Could you check a few things on this model? Use its own coordinates, in mm. Face numbers are marked on the shaded views. Give positions to 0.01 mm unless a question says otherwise; leave off trailing zeros. Loops run counter-clockwise (first coordinate to the right, second up) from the corner with the lowest first, then second, coordinate; pieces in that order, holes last. Notation, with made-up numbers: M 36,76 L 64,76 A19 cw 64,100 Z; hole C 85.5,69 d5. An arc over 180 degrees is marked long. Answer in a Markdown table with one row per item. Add a question column.
Solid Edge part; units mm, degrees
sketch "Sketch1" plane through (0, 0, 0) normal (0, 0, 1) x (1, 0, 0)
  circle A0 centre (0, 0) radius 1.5
extrude "Protrusion1" add sketch "Sketch1" along normal blind 30
sketch "Sketch2" plane through (0, 0, 30) normal (0, 0, 1) x (1, 0, 0)
  circle A0 centre (0, 0) radius 3
extrude "ExtrudedProtrusion_2" add sketch "Sketch2" along normal blind 1.75
chamfer "Chamfer_1" distance 1.75 angle 45 1 edges at (-3, 0, 30)
sketch "Sketch3" plane through (0, 0, 31.75) normal (0, 0, 1) x (0, 1, 0)
  line L0 (0.8978, -1.555) -> (1.7956, 0)
  line L1 (1.7956, 0) -> (0.8978, 1.555)
  line L2 (0.8978, 1.555) -> (-0.8978, 1.555)
  line L3 (-0.8978, 1.555) -> (-1.7956, 0)
  line L4 (-1.7956, 0) -> (-0.8978, -1.555)
  line L5 (-0.8978, -1.555) -> (0.8978, -1.555)
extrude "ExtrudedCutout_1" cut sketch "Sketch3" against normal blind 1
sketch "Sketch4" plane through (0, 0, 0) normal (0, 0, -1) x (0, 1, 0)
  circle A0 centre (0, 0) radius 1.9215
extrude "ExtrudedCutout_2" cut sketch "Sketch4" against normal blind 15.75
properties material "Iron, grey cast type 20"
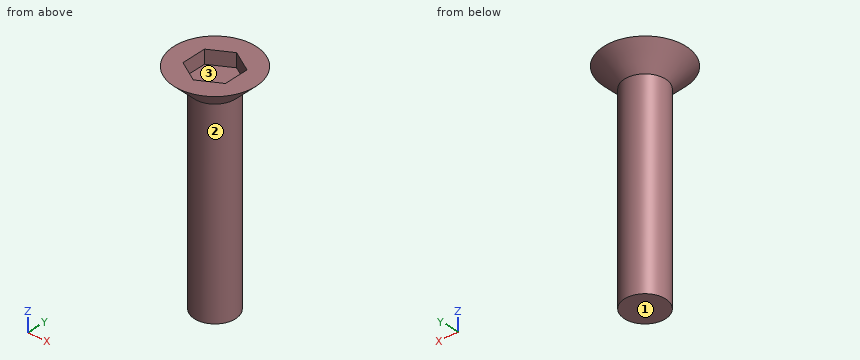
Item 1: Suppose I cut it at A-A (y = 0). List the corners of the cut face in (x, z) for me (3 decimals).
Item 2: If we mould it in two halves opening along Y, with no side actions, what happens to the marked faces 1, 2 and 3? For each: +Y half, -Y half, draft (parallel to the pull), parting line (faces both ways), or undercut.
Item 3: For P1, Ø1.5, axis at x = 2, z = 22, coming from the -Y side; P2, Ø1.5, axis at y = -1.5, z = 20.5, coming from the -X side; P3, Ø0.9, axis at x = 1, y = -0.5, coming from the +Z side, each with a flat end and sliding along its axis, tell me the tip position at first contact or that it passes through.
Item 4: I need wall thicknesses on L1, parallel to Z at x = 0.1, y = -1.3; L2, parallel to Y at x = 1.35, z = 31; L3, parallel to X at y = -0.1, z = 22. Which ranges of each line are inside material? Lowest first, please.
Item 5: Suppose I cut it at B-B (z = 20.25). List the corners of the cut face in (x, y) for me.
Values found:
| question | item | result |
|---|---|---|
| 1 | outline | M -3,31.75 L -1.5,30.25 L -1.5,15.75 L 1.5,15.75 L 1.5,30.25 L 3,31.75 L 1.555,31.75 L 1.555,30.75 L -1.555,30.75 L -1.555,31.75 Z |
| 2 | face 1 | draft |
| 2 | face 2 | parting line |
| 2 | face 3 | undercut |
| 3 | P1 | y = -0.83 |
| 3 | P2 | x = -1.3 |
| 3 | P3 | z = 30.75 |
| 4 | L1 | 15.75 to 30.75 |
| 4 | L2 | -1.8 to -1.02, 1.02 to 1.8 |
| 4 | L3 | -1.5 to 1.5 |
| 5 | outline | C 0,0 d3 |
